```python
from build123d import *

# Parameters (mm, degrees)
F0_R     = 30.353
F1_DEPTH = 31.75
F2_R     = 6.35
F3_DEPTH = 18.415
F4_W     = 9.652
F4_H     = 6.5577
F5_DEPTH = 30.353
F6_R     = 3.379702
F7_DEPTH = 60.706


with BuildPart() as f1:
    # F0 (on Top) → F1 (new body)
    with BuildSketch(Plane.XY):
        Circle(F0_R)
    extrude(amount=F1_DEPTH)

    # F2 (on face) → F3 (cut)
    with BuildSketch(Plane(origin=(0, 0, 0), x_dir=(1, 0, 0), z_dir=(0, 0, -1))):
        Circle(F2_R)
    extrude(amount=-F3_DEPTH, mode=Mode.SUBTRACT)

    # F4 (on Front) → F5 (cut, symmetric)
    with BuildSketch(Plane.XZ):
        Polygon((-4.826, 26.797), (-9.6901, 26.797), (-9.6901, 18.415), (9.6901, 18.415), (9.6901, 26.797), (4.826, 26.797), align=None)
        with Locations((0, 30.07585)):
            Rectangle(F4_W, F4_H)
    extrude(amount=F5_DEPTH, both=True, mode=Mode.SUBTRACT)

    # F6 (on Right) → F7 (cut)
    with BuildSketch(Plane.YZ):
        with Locations((0, 6.477)):
            Circle(F6_R)
    extrude(amount=-F7_DEPTH, mode=Mode.SUBTRACT)


solid = f1.part
```
Could you check a few things on this model? Use its own coordinates, in mm. A direction names the side the tool comes from. Round coordinates to 2 decimals unless told otherwise and drop trailing zeros. Loops run counter-clockwise (first coordinate to the right, second up) from the corner with the lowest first, then second, coordinate; pieces in that order, holes last. Notation, with made-up numbers: M 10.25,69.25 L 35.25,69.25 A26 ccw 35.25,90.25 Z; hole C 83.25,68 d8. An arc over 180 degrees is marked long. Put each result on its own line as item: value.
Q1. On a 3-axis mill with a long thin cutter (end or side, diameter ignored), from which of +Z, -Z, +X, -X, +Y, -Y can I reach the whole of each face in a straight line? I mean faces 4 (the face through (6.057, -1.907, 9.079)), 5 (the face through (4.826, 0, 29)), 6 (the face through (9.69, 0, 23)). Say none if no direction works.
Check result:
face 4: -Z
face 5: +Z, +Y, -Y
face 6: +Y, -Y
Q2. For pin 1 (4 mm diameter, centred on y = 2.5, z = 29, fed in from +X); pin 2 (5 mm diameter, centred on y = -10, z = 22, fed in from +X); pin 3 (5.5 mm diameter, centred on y = 6, z = 28.5, fed in from -X), each with a flat end and sliding along its axis, tell me the tip position at first contact or that it passes through.
Check result:
pin 1: x = 30.35
pin 2: x = 29.41
pin 3: x = -30.18
Q3. Imagine slicing it at C-C (z = 21). Write out the boundary of the cut face in (x, y), then the cut area to 3 significant figures.
Check result:
outline: M -9.69,-28.76 L -9.69,28.76 A30.35 ccw Z; M 9.69,-28.76 A30.35 ccw 9.69,28.76 Z
area: 1,740 mm2
Q4. Imagine slicing it at D-D (z = 17). Write out the boundary of the cut face in (x, y).
Check result:
outline: C 0,0 d60.71; hole C 0,0 d12.7
Q5. Imagine slicing it at A-A (x = 0). Write out the boundary of the cut face in (y, z) (3 decimals), then the cut area to 3 significant figures.
Check result:
outline: M -30.353,0 L -6.35,0 L -6.35,18.415 L -30.353,18.415 Z; M 6.35,0 L 30.353,0 L 30.353,18.415 L 6.35,18.415 Z
area: 884 mm2
Q6. I need wall thicknesses on probe 1 along X at (y, z) = (0, 11.5); probe 2 along Z at (x, y) = (-6.5, -2) (3 decimals). Which ranges of each line are inside material? Lowest first, please.
Check result:
probe 1: -30.35 to -6.35, 6.35 to 30.35
probe 2: 0 to 3.753, 9.201 to 18.415, 26.797 to 31.75
Q7. Imagine slicing it at B-B (y = 0). Write out the boundary of the cut face in (x, z) (3 decimals), then the cut area to 3 significant figures.
Check result:
outline: M -30.353,0 L -6.35,0 L -6.35,3.097 L -30.353,3.097 Z; M -30.353,9.857 L -6.35,9.857 L -6.35,18.415 L -9.69,18.415 L -9.69,26.797 L -4.826,26.797 L -4.826,31.75 L -30.353,31.75 Z; M 4.826,26.797 L 9.69,26.797 L 9.69,18.415 L 6.35,18.415 L 6.35,0 L 30.353,0 L 30.353,31.75 L 4.826,31.75 Z
area: 1,320 mm2
Q8. Thinking about a two-plate mould opening in X: for faces 1 (the face through (28.038, -11.625, 15.653)), 2 (the face through (7, 0, 26.797)), 3 (the face through (-17.691, -0.44, 9.828)), which applies, released by +X, released by -X, zero draft, split by the parting line, or undercut?
Check result:
face 1: split by the parting line
face 2: undercut
face 3: zero draft
